Input: part model. Units: mm. Frame: model coordinates. A direction names the side the tool comes from. Give positions to 0.01 mm unless a question says otherwise; leave off trailing zeros. Write each loop counter-clockwise with the first axis right and the second up, starting at its lowest first coordinate (ties: lowest second). Pieces come first, ordered by that corner, then holes. Notation, with made-up numbers: (-4.75, 13) -> (3.25, 13) arc R4 ccw to (3.25, 20) -> close; hole circle Ø6 at (35, 81.5). An arc over 180 degrees is marked (long way). Return JSON: item names as keys, results as strings. Group by question number.
Item 1: Section C-C, the plane x = 26. Return loops of the section in (y, z).
Item 2: Mould query, pull axis Z, two halves, no side actions, for faces 4 (the face through (0, -32.7, 7)), 5 (the face through (0.41, -32.28, 13)), 6 (the face through (23.6, -0.35, -5.18)). Classes: released by +Z, released by -Z, zero draft, split by the parting line, or undercut.
Item 3: Pin query (flat end, axial travel): P1, Ø0.7, axis at y = -17, z = 12.5, coming from the +X side; P2, Ø6, axis at x = -3.5, y = -14, coming from the -Z side. Return the tip coordinate at first contact, or that it passes through.
Item 4: Set-up query: faces 1 (the face through (23.448, -0.345, 3.597)), 2 (the face through (-31.287, -32.355, 3.451)), 3 (the face through (0, -17, 12.7)). Return all of +Z, -Z, +X, -X, +Y, -Y with unobstructed straight access to the full face (end or side cutting, diameter ignored); none if empty.
Item 5: Section A-A, the plane z = -1.75. Return loops of the section in (x, y), then the cut area to 3 significant figures.
Item 6: Section D-D, the plane x = 11. Return loops of the section in (y, z).
Item 7: Line query: line 1 (X direction, y = -32.3, z = 7.35); line 2 (Y direction, x = -16, z = 11.25); line 3 (Z direction, x = -10.5, y = -11). Output: solid intervals per line, ascending. Write a range as [from, to].
Item 8: Section B-B, the plane z = 7.35. Return loops of the section in (x, y).
from build123d import *

# Parameters (mm, degrees)
SKETCH4_W                    = 64
SKETCH4_H                    = 24
BASE_FLANGE2_DEPTH           = 0.7
CUT_EXTRUDE1_REACH           = 36.183
SKETCH7_W                    = 41
SKETCH7_H                    = 21
CUT_EXTRUDE2_REACH           = 36.183
SKETCH8_R                    = 1.7
EDGE_FLANGE1_DEPTH           = 59
EDGE_FLANGE2_STRIP_W         = 4.2
EDGE_FLANGE2_STRIP_H         = 0.7
EDGE_FLANGE2_STRIP_CUT_DEPTH = 59
EDGE_FLANGE2_DEPTH           = 59
SKETCH16_W                   = 2.5
SKETCH16_H                   = 9.3
TAB1_DEPTH                   = 0.7
CUT_EXTRUDE3_REACH           = 49.197
SKETCH15_R                   = 1.7
BREAK_CORNER1_START          = -32.7
BREAK_CORNER1_DEPTH          = 32.7
BREAK_CORNER1_2_DEPTH        = 0.7


# Read off the part's stored shape, not the designer's step: Break-Corner1
# Sheet-metal steps are written as plain solids
with BuildPart() as part:
    # Sketch4 → Base-Flange2 (new body)
    with BuildSketch(Plane(origin=(0, 0, 0), x_dir=(1, 0, 0), z_dir=(0, 1, 0))):
        Rectangle(SKETCH4_W, SKETCH4_H)
    extrude(amount=-BASE_FLANGE2_DEPTH)

    # Sketch7 → Cut-Extrude1 (cut, up to next)
    with BuildSketch(Plane(origin=(0, 0, 0), x_dir=(1, 0, 0), z_dir=(0, 1, 0)), mode=Mode.PRIVATE) as cut_extrude1_sk1:
        with Locations((0, 1.5)):
            Rectangle(SKETCH7_W, SKETCH7_H)
    cut_extrude1_tool1 = extrude(cut_extrude1_sk1.sketch, amount=-CUT_EXTRUDE1_REACH, mode=Mode.PRIVATE) & part.part
    add(cut_extrude1_tool1.solids().sort_by_distance((0, 0, -1.5))[0], mode=Mode.SUBTRACT)

    # Sketch8 → Cut-Extrude2 (cut, up to next)
    with BuildSketch(Plane(origin=(0, 0, 0), x_dir=(1, 0, 0), z_dir=(0, 1, 0)), mode=Mode.PRIVATE) as cut_extrude2_sk1:
        with Locations(Location((-25.108, -3.9655, 0), (0, 0, 270))):
            Circle(SKETCH8_R)
    cut_extrude2_tool1 = extrude(cut_extrude2_sk1.sketch, amount=-CUT_EXTRUDE2_REACH, mode=Mode.PRIVATE) & part.part
    # Sketch8 → Cut-Extrude2 (cut, up to next)
    with BuildSketch(Plane(origin=(0, 0, 0), x_dir=(1, 0, 0), z_dir=(0, 1, 0)), mode=Mode.PRIVATE) as cut_extrude2_sk2:
        with Locations(Location((-25.108, 5.9655, 0), (0, 0, 270))):
            Circle(SKETCH8_R)
    cut_extrude2_tool2 = extrude(cut_extrude2_sk2.sketch, amount=-CUT_EXTRUDE2_REACH, mode=Mode.PRIVATE) & part.part
    # Sketch8 → Cut-Extrude2 (cut, up to next)
    with BuildSketch(Plane(origin=(0, 0, 0), x_dir=(1, 0, 0), z_dir=(0, 1, 0)), mode=Mode.PRIVATE) as cut_extrude2_sk3:
        with Locations(Location((25.108, -3.9655, 0), (0, 0, 270))):
            Circle(SKETCH8_R)
    cut_extrude2_tool3 = extrude(cut_extrude2_sk3.sketch, amount=-CUT_EXTRUDE2_REACH, mode=Mode.PRIVATE) & part.part
    # Sketch8 → Cut-Extrude2 (cut, up to next)
    with BuildSketch(Plane(origin=(0, 0, 0), x_dir=(1, 0, 0), z_dir=(0, 1, 0)), mode=Mode.PRIVATE) as cut_extrude2_sk4:
        with Locations(Location((25.108, 5.9655, 0), (0, 0, 270))):
            Circle(SKETCH8_R)
    cut_extrude2_tool4 = extrude(cut_extrude2_sk4.sketch, amount=-CUT_EXTRUDE2_REACH, mode=Mode.PRIVATE) & part.part
    add(cut_extrude2_tool1.solids().sort_by_distance((-25.108, 0, 3.9655))[0], mode=Mode.SUBTRACT)
    add(cut_extrude2_tool2.solids().sort_by_distance((-25.108, 0, -5.9655))[0], mode=Mode.SUBTRACT)
    add(cut_extrude2_tool3.solids().sort_by_distance((25.108, 0, 3.9655))[0], mode=Mode.SUBTRACT)
    add(cut_extrude2_tool4.solids().sort_by_distance((25.108, 0, -5.9655))[0], mode=Mode.SUBTRACT)

    # Edge-Flange1 section (across the edge) → Edge-Flange1 (add)
    with BuildSketch(Plane(origin=(29.5, -0.7, 12.7), x_dir=(0, 0, -1), z_dir=(-1, 0, 0))):
        with BuildLine():
            Line((-0.7, 0.7), (-0.7, 32))
            Line((-0.7, 32), (0, 32))
            Line((0, 32), (0, 0.7))
            ThreePointArc((0, 0.7), (0.205025253, 0.205025253), (0.7, 0))
            Line((0.7, 0), (0.7, -0.7))
            ThreePointArc((0.7, -0.7), (-0.289949494, -0.289949494), (-0.7, 0.7))
        make_face()
    extrude(amount=EDGE_FLANGE1_DEPTH)

    # Edge-Flange2 strip (across the edge) → Edge-Flange2 strip cut (cut)
    with BuildSketch(Plane(origin=(29.5, -32.7, 12.7), x_dir=(0, 1, 0), z_dir=(-1, 0, 0))):
        with Locations((-0.7, -0.35)):
            Rectangle(EDGE_FLANGE2_STRIP_W, EDGE_FLANGE2_STRIP_H)
    extrude(amount=EDGE_FLANGE2_STRIP_CUT_DEPTH, mode=Mode.SUBTRACT)

    # Edge-Flange2 section (across the edge) → Edge-Flange2 (add)
    with BuildSketch(Plane(origin=(29.5, -32.7, 12.7), x_dir=(0, 1, 0), z_dir=(-1, 0, 0))):
        with BuildLine():
            Line((0, 0.7), (0, 10))
            Line((0, 10), (0.7, 10))
            Line((0.7, 10), (0.7, 0.7))
            ThreePointArc((0.7, 0.7), (0.905025253, 0.205025253), (1.4, 0))
            Line((1.4, 0), (1.4, -0.7))
            ThreePointArc((1.4, -0.7), (0.410050506, -0.289949494), (0, 0.7))
        make_face()
    extrude(amount=EDGE_FLANGE2_DEPTH)

    # Sketch16 → Tab1 (add)
    with BuildSketch(Plane(origin=(0, -32, 0), x_dir=(1, 0, 0), z_dir=(0, 1, 0))):
        with Locations((-30.75, -7.35)):
            Rectangle(SKETCH16_W, SKETCH16_H)
        with Locations((30.75, -7.35)):
            Rectangle(SKETCH16_W, SKETCH16_H)
    extrude(amount=-TAB1_DEPTH)

    # Sketch15 → Cut-Extrude3 (cut, up to next)
    with BuildSketch(Plane(origin=(0, -32, 0), x_dir=(1, 0, 0), z_dir=(0, 1, 0)), mode=Mode.PRIVATE) as cut_extrude3_sk1:
        with Locations(Location((25, -7.35, 0), (0, 0, 270))):
            Circle(SKETCH15_R)
    cut_extrude3_tool1 = extrude(cut_extrude3_sk1.sketch, amount=-CUT_EXTRUDE3_REACH, mode=Mode.PRIVATE) & part.part
    # Sketch15 → Cut-Extrude3 (cut, up to next)
    with BuildSketch(Plane(origin=(0, -32, 0), x_dir=(1, 0, 0), z_dir=(0, 1, 0)), mode=Mode.PRIVATE) as cut_extrude3_sk2:
        with Locations(Location((-25, -7.35, 0), (0, 0, 90))):
            Circle(SKETCH15_R)
    cut_extrude3_tool2 = extrude(cut_extrude3_sk2.sketch, amount=-CUT_EXTRUDE3_REACH, mode=Mode.PRIVATE) & part.part
    add(cut_extrude3_tool1.solids().sort_by_distance((25, -32, 7.35))[0], mode=Mode.SUBTRACT)
    add(cut_extrude3_tool2.solids().sort_by_distance((-25, -32, 7.35))[0], mode=Mode.SUBTRACT)

    # Break-Corner1 outline → Break-Corner1 (cut)
    with BuildSketch(Plane(origin=(0, 0, 0), x_dir=(1, 0, 0), z_dir=(0, 1, 0)).offset(BREAK_CORNER1_START)):
        with BuildLine():
            Line((-32, 12), (-32, 9.501))
            ThreePointArc((-32, 9.501), (-31.268059846, 11.268059846), (-29.501, 12))
            Line((-29.501, 12), (-32, 12))
        make_face()
        with BuildLine():
            ThreePointArc((29.501, 12), (31.268059846, 11.268059846), (32, 9.501))
            Line((32, 9.501), (32, 12))
            Line((32, 12), (29.501, 12))
        make_face()
        with BuildLine():
            Line((32, -12), (32, -9.501))
            ThreePointArc((32, -9.501), (31.268059846, -11.268059846), (29.501, -12))
            Line((29.501, -12), (32, -12))
        make_face()
        with BuildLine():
            ThreePointArc((-29.501, -12), (-31.268059846, -11.268059846), (-32, -9.501))
            Line((-32, -9.501), (-32, -12))
            Line((-32, -12), (-29.501, -12))
        make_face()
    extrude(amount=BREAK_CORNER1_DEPTH, mode=Mode.SUBTRACT)

    # Break-Corner1 2 outline → Break-Corner1 2 (cut)
    with BuildSketch(Plane(origin=(0, 0, 0), x_dir=(1, 0, 0), z_dir=(0, 1, 0)).offset(BREAK_CORNER1_START)):
        with BuildLine():
            Line((32, -2.7), (29.501, -2.7))
            ThreePointArc((29.501, -2.7), (31.268059846, -3.431940154), (32, -5.199))
            Line((32, -5.199), (32, -2.7))
        make_face()
        with BuildLine():
            Line((-32, -2.7), (-32, -5.199))
            ThreePointArc((-32, -5.199), (-31.268059846, -3.431940154), (-29.501, -2.7))
            Line((-29.501, -2.7), (-32, -2.7))
        make_face()
    extrude(amount=BREAK_CORNER1_2_DEPTH, mode=Mode.SUBTRACT)


solid = part.part
Answer below:
{
 "1": {"outline": "(-32.7, 2.7) -> (-32, 2.7) -> (-32, 5.98) -> (-32.7, 5.98) -> close; (-32.7, 8.72) -> (-32, 8.72) -> (-32, 12) arc R0.7 cw to (-31.3, 12.7) -> (-1.4, 12.7) arc R0.7 cw to (-0.7, 12) -> (-0.7, 5.41) -> (0, 5.41) -> (0, 12) arc R1.4 ccw to (-1.4, 13.4) -> (-31.3, 13.4) arc R1.4 ccw to (-32.7, 12) -> close; (-0.7, -12) -> (0, -12) -> (0, -7.41) -> (-0.7, -7.41) -> close; (-0.7, -4.52) -> (0, -4.52) -> (0, 2.52) -> (-0.7, 2.52) -> close"},
 "2": {"face 4": "zero draft", "face 5": "released by +Z", "face 6": "undercut"},
 "3": {"P1": "stops at x = 29.5", "P2": "stops at z = 12.7"},
 "4": {"face 1": "+Y", "face 2": "-Z, -X, -Y", "face 3": "-Z, +X, -X"},
 "5": {"outline": "(-32, -0.7) -> (-20.5, -0.7) -> (-20.5, 0) -> (-32, 0) -> close; (20.5, -0.7) -> (32, -0.7) -> (32, 0) -> (20.5, 0) -> close", "area": "16.1 mm2"},
 "6": {"outline": "(-32.7, 2.7) -> (-32, 2.7) -> (-32, 12) arc R0.7 cw to (-31.3, 12.7) -> (-1.4, 12.7) arc R0.7 cw to (-0.7, 12) -> (-0.7, 9) -> (0, 9) -> (0, 12) arc R1.4 ccw to (-1.4, 13.4) -> (-31.3, 13.4) arc R1.4 ccw to (-32.7, 12) -> close"},
 "7": {"line 1": "x = [-32, -26.7], [-23.3, 23.3], [26.7, 32]", "line 2": "y = [-32.7, -32], [-0.7, 0]", "line 3": "z = [12.7, 13.4]"},
 "8": {"outline": "(-32, -32.7) -> (-26.7, -32.7) -> (-26.7, -32) -> (-32, -32) -> close; (-32, -0.7) -> (-20.5, -0.7) -> (-20.5, 0) -> (-32, 0) -> close; (-23.3, -32.7) -> (23.3, -32.7) -> (23.3, -32) -> (-23.3, -32) -> close; (20.5, -0.7) -> (32, -0.7) -> (32, 0) -> (20.5, 0) -> close; (26.7, -32.7) -> (32, -32.7) -> (32, -32) -> (26.7, -32) -> close"}
}
